Read the model definition and answer for the solid it produces. Units are mm, in the model's axes. A direction names the side the tool comes from. Coordinates: 2 decimals unless noted, no trailing zeros. Write each loop counter-clockwise with the first axis right and the second up, starting at its lowest first coordinate (ties: lowest second). Pieces come first, ordered by that corner, then holes. Notation, with made-up numbers: (48.5, -16.75) - (65.5, -16.75) arc R15 ccw to (65.5, 9.25) - close; hole circle Ø7 at (24, 35.25). An arc over 180 degrees is marked (long way). Use a Markdown table: item, result.
from build123d import *

# Parameters (mm, degrees)
F0_R            = 52.5
F1_DEPTH        = 18
F2_R            = 45.125
F3_DEPTH        = 9
F4_SIZE         = 1
F5_R            = 9.5
F6_DEPTH        = 27
F7_R            = 5
F8_DEPTH        = 11
F9_SIZE2        = 0.5773502692
F9_SIZE         = 1
F11_D           = 11
F11_CBORE_D     = 18
F11_CBORE_DEPTH = 4


with BuildPart() as f1:
    # F0 (on Right) → F1 (new body)
    with BuildSketch(Plane.YZ):
        Circle(F0_R)
    extrude(amount=-F1_DEPTH)

    # F2 (on face) → F3 (cut)
    with BuildSketch(Plane(origin=(-18, 0, 0), x_dir=(0, -1, 0), z_dir=(-1, 0, 0))):
        Circle(F2_R)
    extrude(amount=-F3_DEPTH, mode=Mode.SUBTRACT)

    # F4
    f4_edges = [f1.edges().sort_by_distance(p)[0] for p in [
        (-18, -52.5, 0),
        (-18, 45.125, 0),
    ]]
    chamfer(f4_edges, length=F4_SIZE)

    # F5 (on face) → F6 (join)
    with BuildSketch(Plane.YZ):
        Circle(F5_R)
    extrude(amount=F6_DEPTH)

    # F7 (on face) → F8 (join)
    with BuildSketch(Plane.YZ.offset(27)):
        Circle(F7_R)
    extrude(amount=F8_DEPTH)

    # F9
    f9_edges = [f1.edges().sort_by_distance(p)[0] for p in [
        (38, -5, 0),
    ]]
    f9_side = f1.faces().sort_by_distance((32.5, -5, 0))[0]
    chamfer(f9_edges, length=F9_SIZE, length2=F9_SIZE2, reference=f9_side)

    # F11 (through all)
    with Locations(Plane.YZ):
        with Locations((0, -22.5), (0, 22.5)):
            CounterBoreHole(F11_D / 2, F11_CBORE_D / 2, F11_CBORE_DEPTH)


solid = f1.part
(1) A cutting plane is placed at C-C, the plane x = 16. Write down the section's boundary in (y, z), and give its area (3 significant figures).
Report:
| item | result |
|---|---|
| outline | circle Ø19 at (0, 0) |
| area | 284 mm² |
(2) For faces 4 (the cylindrical face through (-13.06, 35.81, -27.46)), 5 (the flat face through (-4, -4.1, 18.6)), 6 (the cylindrical face through (-6.535, 0.716, 27.953)), determine the directions among +Z, -Z, +X, -X, +Y, -Y from which every point of the face is accessible in a straight line to the end or side of a thin tool.
Report:
| item | result |
|---|---|
| face 4 | -X |
| face 5 | +X |
| face 6 | +X, -X |
(3) A cutting plane is placed at D-D, the plane x = -6. Write down the section's boundary in (y, z).
Report:
| item | result |
|---|---|
| outline | circle Ø105 at (0, 0); hole circle Ø11 at (0, -22.5); hole circle Ø11 at (0, 22.5) |
(4) Straight lines are drawn through the part: L1, parallel to Z at x = -1.75, y = 0; L2, parallel to Z at x = -6, y = 0; L3, parallel to Z at x = -11.75, y = 0 (3 decimals). For each, find the intervals that lie inside material, in ascending order.
Report:
| item | result |
|---|---|
| L1 | z = -52.5 to -31.5, -13.5 to 13.5, 31.5 to 52.5 |
| L2 | z = -52.5 to -28, -17 to 17, 28 to 52.5 |
| L3 | z = -52.5 to -45.125, 45.125 to 52.5 |
(5) The mould has two halves that part along Y. Classify faces 1 (the flat face through (38, 0, 0)), 2 (the flat face through (-4, -4.1, -26.4)), 3 (the cylindrical face through (-8.381, 50.076, 15.77)): pulls with the +Y half, pulls with the -Y half, needs draft (parallel to the pull), parting line crosses it, or undercut.
Report:
| item | result |
|---|---|
| face 1 | needs draft |
| face 2 | undercut |
| face 3 | parting line crosses it |
(6) A cutting plane is placed at B-B, the plane y = 0. Count the separate pieces of the cut face and the enclosed holes in it, and give its area (3 significant figures).
Report:
| item | result |
|---|---|
| separate pieces | 3 |
| enclosed holes | 0 |
| area | 1,440 mm² |
(7) A cutting plane is placed at A-A, the plane z = 0. Write down the section's boundary in (x, y) (3 decimals).
Report:
| item | result |
|---|---|
| outline | (-18, -51.5) - (-17, -52.5) - (0, -52.5) - (0, -9.5) - (27, -9.5) - (27, -5) - (37, -5) - (38, -4.423) - (38, 4.423) - (37, 5) - (27, 5) - (27, 9.5) - (0, 9.5) - (0, 52.5) - (-17, 52.5) - (-18, 51.5) - (-18, 46.125) - (-17, 45.125) - (-9, 45.125) - (-9, -45.125) - (-17, -45.125) - (-18, -46.125) - close |
(8) Each of these flat-tipped pins is pushed along its axis until it touches: P1, Ø4, axis at y = -4, z = 12, coming from the +X side; P2, Ø10, axis at x = 27.5, y = 18.5, coming from the -Z side; P3, Ø8, axis at y = 11, z = 3.5, coming from the -X side; P4, Ø9, axis at y = 2.5, z = -19.5, coming from the +X side. Where does it stop, or does it pass through?
Report:
| item | result |
|---|---|
| P1 | stops at x = 0 |
| P2 | passes through |
| P3 | stops at x = -9 |
| P4 | stops at x = -4 |
